Source: three-view drawing plus pictorial views. Frame: mm from the lowest corner of the part. A direction names the side the tool comes from. Give positions to 0.01 mm unless a question says otherwise; leave off trailing zeros. Write each loop counter-clockwise with the first axis right and the second up, starting at its lowest first coordinate (ties: lowest second). Pieces come first, ordered by that corner, then holes.
Q1. Reachability of the marked faces 1, 2 and 3 from +Z, -Z, +X, -X, +Y, -Y: full face, straight path, thin tool, end or side. Return the list, or none.
Q2. Cut plane C-C on z = 1.65. Return the cut outline in (x, y).
Q3. Line query: L1, parallel to Y at x = 25.6, z = 2.1; L2, parallel to Z at x = 5.5, y = 16; L3, parallel to X at y = 9, z = 3.25. Output: solid intervals per line, ascending.
Q4. Cut plane D-D on x = 16.75. Return the cut outline in (y, z).
Q5. Cut plane B-B on y = 12.5. Return the cut outline in (x, z).
Q6. Pin query (flat end, axial travel): pin 1 (9.5 mm diameter, centred on x = 13, y = 6.5, fed in from +Z); pin 2 (1.5 mm diameter, centred on y = 2.5, z = 1.5, fed in from -X) (1 decimal); pin 3 (2.5 mm diameter, centred on y = 9.5, z = 2.1, fed in from -X); pin 4 (1.6 mm diameter, centred on y = 9.5, z = 3, fed in from -X). Return the tip coordinate at first contact, or that it passes through.
Q7. Cut plane A-A on z = 0.4. Return the cut outline in (x, y).
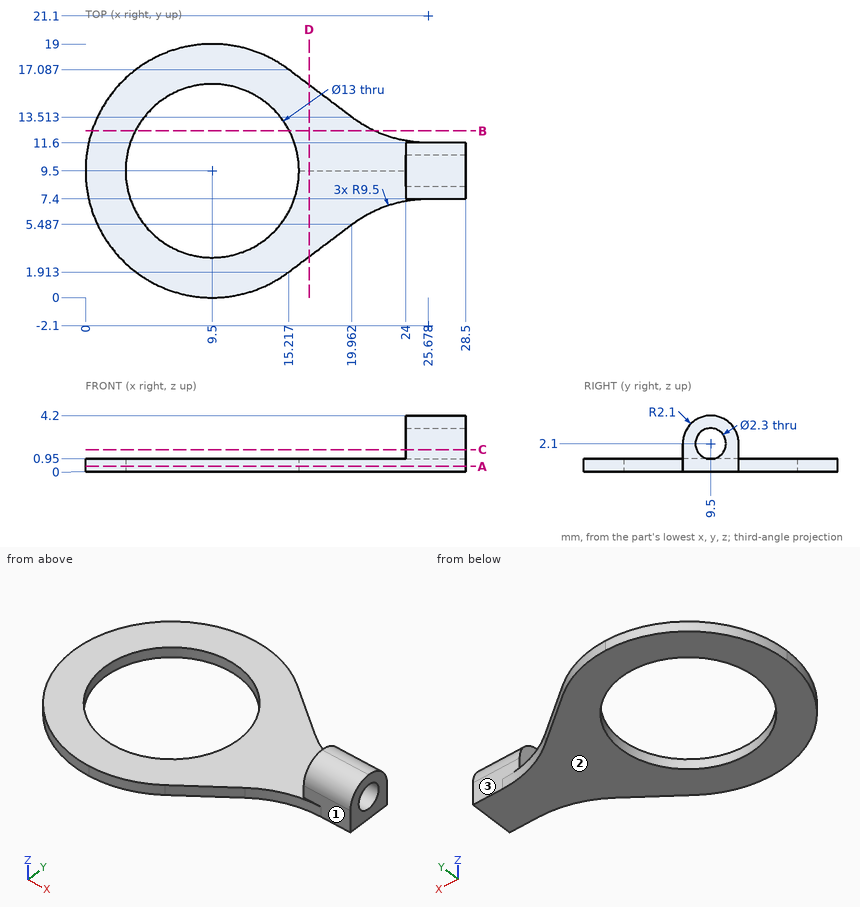
Data:
1. face 1: +Z, +X, -Y
1. face 2: -Z, +X, -X, +Y, -Y
1. face 3: +Z, +X, +Y
2. outline: (24, 7.4) - (28.5, 7.4) - (28.5, 8.44) - (24, 8.44) - close; (24, 10.56) - (28.5, 10.56) - (28.5, 11.6) - (24, 11.6) - close
3. L1: y = 7.4 to 8.35, 10.65 to 11.6
3. L2: z = 0 to 0.95
3. L3: x = 24 to 28.5
4. outline: (3.07, 0) - (15.93, 0) - (15.93, 0.95) - (3.07, 0.95) - close
5. outline: (0.49, 0) - (3.73, 0) - (3.73, 0.95) - (0.49, 0.95) - close; (15.27, 0) - (21.64, 0) - (21.64, 0.95) - (15.27, 0.95) - close
6. pin 1: stops at z = 0.95
6. pin 2: stops at x = 2.6
6. pin 3: stops at x = 0
6. pin 4: stops at x = 24
7. outline: (15.22, 1.91) - (19.96, 5.49) arc R9.5 cw to (25.68, 7.4) - (28.5, 7.4) - (28.5, 11.6) - (25.68, 11.6) arc R9.5 cw to (19.96, 13.51) - (15.22, 17.09) arc R9.5 ccw (long way) to start; hole circle Ø13 at (9.5, 9.5)
